Read the model definition and answer for the solid it produces. Units are mm, in the model's axes. A direction names the side the tool comes from. Coordinates: 2 decimals unless noted, no trailing zeros. Order: outer loops, then holes, each group sorted by start corner. A loop starts at its lowest first (then second) coordinate and runs counter-clockwise, first axis right, second up. Notation, with made-up numbers: (17.25, 73.5) - (75.25, 73.5) arc R15 cw to (75.25, 82.5) - close; hole circle Ø1 at (-17, 64.5). An arc over 180 degrees is marked (long way). Answer as a JSON object with one key per item and string values. Group by question number.
Autodesk Inventor part; units mm, degrees
ref_plane "YZ Plane" through (0, 0, 0) normal (1, 0, 0) x (0, 1, 0)
ref_plane "XZ Plane" through (0, 0, 0) normal (0, 1, 0) x (-1, 0, 0)
ref_plane "XY Plane" through (0, 0, 0) normal (0, 0, 1) x (1, 0, 0)
sketch "Boceto3" plane through (0, 0, 0) normal (0, 0, 1) x (1, 0, 0)
  line L0 (-53.34, 0) -> (53.34, 0) construction
  line L1 (0, -53.34) -> (0, 53.34) construction
  line L2 (0, -25.4) -> (25.4, 0) construction
  line L3 (25.4, 0) -> (0, 25.4) construction
  line L4 (0, 25.4) -> (-25.4, 0) construction
  line L5 (-25.4, 0) -> (0, -25.4) construction
  line L6 (0, -25.4) -> (0, 25.4) construction
  line L7 (25.4, 0) -> (-25.4, 0) construction
  arc A0 (-34.3803, 8.9803) -> (-34.3803, -8.9803) centre (-25.4, 0) ccw
  arc A1 (8.9803, 34.3803) -> (-8.9803, 34.3803) centre (0, 25.4) ccw
  arc A2 (34.3803, -8.9803) -> (34.3803, 8.9803) centre (25.4, 0) ccw
  arc A3 (-8.9803, -34.3803) -> (8.9803, -34.3803) centre (0, -25.4) ccw
  circle A4 centre (-25.4, 0) radius 4.3688
  circle A5 centre (0, 25.4) radius 4.3688
  circle A6 centre (25.4, 0) radius 4.3688
  circle A7 centre (0, -25.4) radius 4.3688
  line L8 (-34.3803, 8.9803) -> (-8.9803, 34.3803)
  line L9 (8.9803, 34.3803) -> (34.3803, 8.9803)
  line L10 (34.3803, -8.9803) -> (8.9803, -34.3803)
  line L11 (-8.9803, -34.3803) -> (-34.3803, -8.9803)
  point P0 (0, 0)
  dimension "d30" = 25.4
  dimension "d31" = 50.8
  dimension "d32" = 50.8
  dimension "d33" = 25.4
  dimension "d34" = 12.7
  dimension "d35" = 12.7
  dimension "d36" = 12.7
  dimension "d37" = 12.7
  dimension "d38" = 8.7376
  dimension "d39" = 8.7376
  dimension "d40" = 8.7376
  dimension "d41" = 8.7376
extrude "Base" add sketch "Boceto3" along normal blind 10.16
sketch "Boceto4" plane through (0, 0, 10.16) normal (0, 0, 1) x (1, 0, 0)
  circle A0 centre (0, 0) radius 13.97
  dimension "d44" = 27.94
extrude "Cilindro" add sketch "Boceto4" along normal blind 55.88
sketch "Boceto5" plane through (0, 0, 66.04) normal (0, 0, 1) x (1, 0, 0)
  line L0 (-25.4, -25.4) -> (25.4, -25.4) construction
  line L1 (25.4, -25.4) -> (25.4, 25.4) construction
  line L2 (25.4, 25.4) -> (-25.4, 25.4) construction
  line L3 (-25.4, 25.4) -> (-25.4, -25.4) construction
  line L4 (-25.4, -25.4) -> (25.4, 25.4) construction
  line L5 (25.4, -25.4) -> (-25.4, 25.4) construction
  arc A0 (-19.05, 36.3985) -> (-36.3985, 19.05) centre (-25.4, 25.4) ccw
  arc A1 (-36.3985, -19.05) -> (-19.05, -36.3985) centre (-25.4, -25.4) ccw
  arc A2 (19.05, -36.3985) -> (36.3985, -19.05) centre (25.4, -25.4) ccw
  arc A3 (36.3985, 19.05) -> (19.05, 36.3985) centre (25.4, 25.4) ccw
  circle A4 centre (-25.4, 25.4) radius 5.1562
  circle A5 centre (-25.4, -25.4) radius 5.1562
  circle A6 centre (25.4, -25.4) radius 5.1562
  circle A7 centre (25.4, 25.4) radius 5.1562
  arc A8 (-36.3985, -19.05) -> (-36.3985, 19.05) centre (-69.3941, 0) ccw
  arc A9 (-19.05, 36.3985) -> (19.05, 36.3985) centre (0, 69.3941) ccw
  arc A10 (36.3985, 19.05) -> (36.3985, -19.05) centre (69.3941, 0) ccw
  arc A11 (19.05, -36.3985) -> (-19.05, -36.3985) centre (0, -69.3941) ccw
  point P0 (0, 0)
  dimension "d47" = 50.8
  dimension "d48" = 50.8
  dimension "d49" = 25.4
  dimension "d50" = 25.4
  dimension "d51" = 25.4
  dimension "d52" = 25.4
  dimension "d53" = 10.3124
  dimension "d54" = 10.3124
  dimension "d55" = 10.3124
  dimension "d56" = 10.3124
  dimension "d57" = 25.4
  dimension "d58" = 76.2
  dimension "d59" = 76.2
  dimension "d60" = 76.2
  dimension "d61" = 76.2
extrude "Extrusión5" add sketch "Boceto5" against normal blind 12.7
sketch "Boceto6" plane through (0, 0, 66.04) normal (0, 0, 1) x (1, 0, 0)
  point P0 (0, 0)
  point P1 (0, 0)
hole "Agujero1" at (0, 0, 66.04) direction (0, 0, -1) diameter 19.05 depth 38.1 counterbore diameter 38.1 counterbore depth 2.54
draft "Cara para el ángulo de desmoldeo1" angle 45 pull direction (0, 0, 1) faces at (1.5329, -18.9882, 65.1933) fixed edges at (0, 19.05, 66.04)
fillet "Empalme1" radius 1.524 17 edges at (0, 38.1, 10.16) (-21.6803, 21.6803, 10.16) (-38.1, 0, 10.16) (-21.6803, -21.6803, 10.16) (0, -38.1, 10.16) (21.6803, -21.6803, 10.16) (38.1, 0, 10.16) (21.6803, 21.6803, 10.16) (-13.97, 0, 10.16) (34.3803, 34.3803, 53.34) (31.2941, 0, 53.34) (34.3803, -34.3803, 53.34) (0, -31.2941, 53.34) (-34.3803, -34.3803, 53.34) (-31.2941, 0, 53.34) (-34.3803, 34.3803, 53.34) (0, 31.2941, 53.34)
properties part number "Lab6A01209499P2"
1. For a pull along Z with two mould halves and no side action, classify faces 4 (the cylindrical face through (5.796, 7.559, 45.471)), 5 (the flat face through (-1, 1, 0)), 6 (the flat face through (16, 1, 10.16)) as pulls with the +Z half, pulls with the -Z half, needs draft (parallel to the pull), parting line crosses it, or undercut.
2. A cutting plane is placed at C-C on z = 34. Write down the section's boundary in (x, y) (3 decimals).
3. A cutting plane is placed at A-A on z = 56. State how many separate pieces and enclosed holes the cut face has, and give its area (3 significant figures).
4. For faces 1 (the cylindrical face through (-1.82, -13.85, 32.22)), 2 (the cylindrical face through (-21.364, 1.673, 5.009)), 3 (the flat face through (21.5, 21.86, 4.26)), determine the directions among +Z, -Z, +X, -X, +Y, -Y from which every point of the face is accessible in a straight line to the end or side of a thin tool.
5. Given pin 1 (11.5 mm diameter, centred on x = 0, y = 0, fed in from +Z); pin 2 (21 mm diameter, centred on x = -2.5, y = 1.5, fed in from +Z); pin 3 (5 mm diameter, centred on x = 0, y = -25.4, fed in from -Z); pin 4 (6 mm diameter, centred on y = -20.5, z = 15.5, fed in from +X), each flat-ended and moving along its own axis, determine where each tip first touches the part or whether it passes through.
6. Straight lines are drawn through the part: L1, parallel to Y at x = -25.4, z = 59; L2, parallel to Y at x = 0, z = 2; L3, parallel to X at y = 25, z = 61. For each, find the intervals that lie inside material, in ascending order.
Derived:
{
 "1": {"face 4": "needs draft", "face 5": "pulls with the -Z half", "face 6": "undercut"},
 "2": {"outline": "circle Ø27.94 at (0, 0); hole circle Ø19.05 at (0, 0)"},
 "3": {"separate pieces": "1", "enclosed holes": "5", "area": "4,240 mm2"},
 "4": {"face 1": "none", "face 2": "-Z", "face 3": "-Z, +X, +Y"},
 "5": {"pin 1": "stops at z = 27.94", "pin 2": "stops at z = 63.5", "pin 3": "stops at z = 53.34", "pin 4": "passes through"},
 "6": {"L1": "y = -38.1 to -30.56, -20.24 to 20.24, 30.56 to 38.1", "L2": "y = -38.1 to -29.77, -21.03 to 21.03, 29.77 to 38.1", "L3": "x = -38.09 to -30.54, -20.26 to 20.26, 30.54 to 38.09"}
}
